For this review, use the dimensioned drawing (mm, ordinates from the lowest corner) and the shaded views. Give positions to 0.01 mm unless a question says otherwise; leave off trailing zeros. Loops run counter-clockwise (first coordinate to the right, second up) from the corner with the lowest first, then second, coordinate; pieces in that order, holes last. Notation, with made-up numbers: (37.25, 76) -> (84.25, 76) arc R15 cw to (84.25, 84) -> close; hole circle Ø1 at (-17, 1.25). An arc over 180 degrees is marked (long way). Write each question's results on one line, items separated by ' | '. Start each with the question number.
Q1. Wall thickness on L1, parallel to X at y = 11.5, z = 255; L2, parallel to Z at x = 41, y = 5.25; L3, parallel to Z at x = 40, y = 4.5: over which ranges is each line inside the solid? List them lowest first. Write a range as [from, to].
Q2. We need section A-A (z = 255). Write out the cut boundary in (x, y).
Q3. Insertion check: pin 1 Ø9.5 at (x, z) = (40, 40) entering from +Y. The pin has a flat end and moves straight along its axis. Give the tip position at first contact, or say it passes through.
Q4. We need section B-B (x = 247). Write out the cut boundary in (y, z).
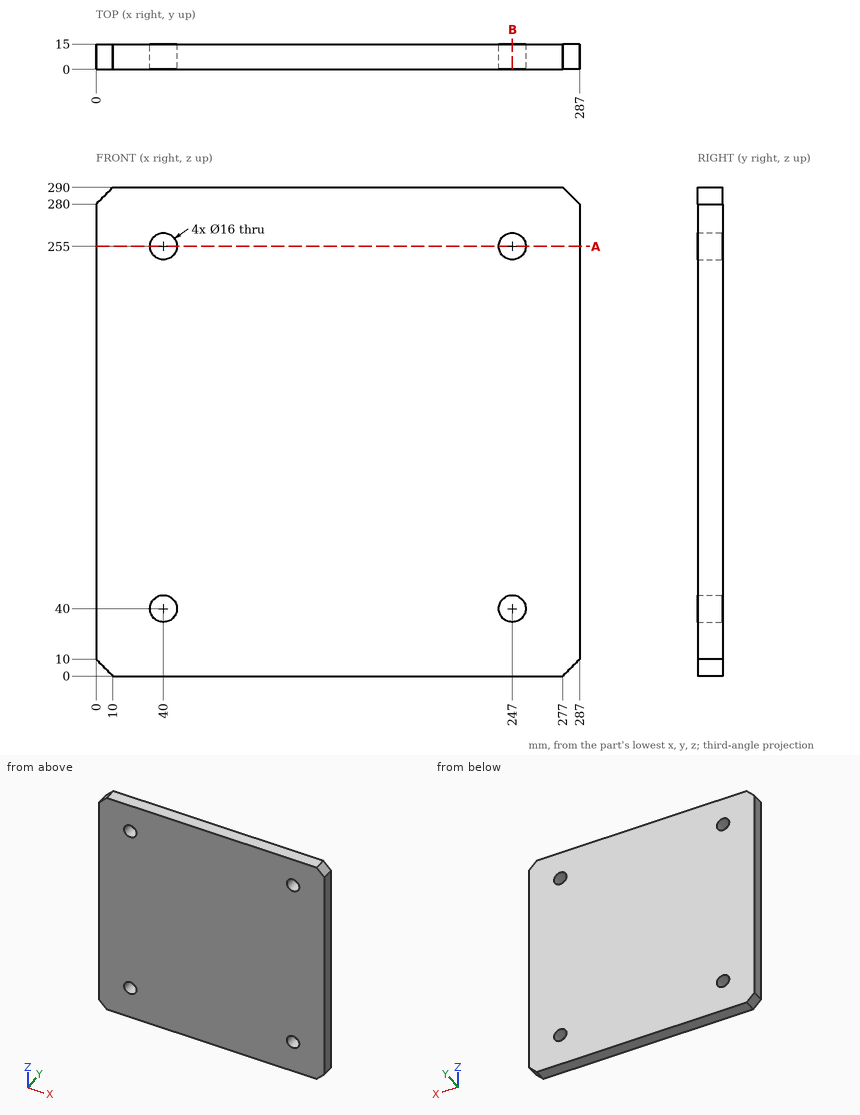
Output:
1) L1: [0, 32], [48, 239], [255, 287] | L2: [0, 32.06], [47.94, 247.06], [262.94, 290] | L3: [0, 32], [48, 247], [263, 290]
2) outline: (0, 0) -> (32, 0) -> (32, 15) -> (0, 15) -> close; (48, 0) -> (239, 0) -> (239, 15) -> (48, 15) -> close; (255, 0) -> (287, 0) -> (287, 15) -> (255, 15) -> close
3) pin 1: through
4) outline: (0, 0) -> (15, 0) -> (15, 32) -> (0, 32) -> close; (0, 48) -> (15, 48) -> (15, 247) -> (0, 247) -> close; (0, 263) -> (15, 263) -> (15, 290) -> (0, 290) -> close
